For this review, take the finished solid that the model builds, in its own axes (mm). A direction names the side the tool comes from. Give positions to 0.01 mm unless a question says otherwise; leave off trailing zeros. Loops run counter-clockwise (first coordinate to the right, second up) from the corner with the lowest first, then second, coordinate; pieces in that order, holes last. Notation, with made-up numbers: M 65,23.5 L 92,23.5 A32 ccw 92,62.5 Z; hole C -38.75,35.5 d8. An arc over 180 degrees is marked long. Use CSV: the item, a comma, the result in double quotes. Start each with the question number.
1. To check wall thickness, follow line 1 (Y direction, x = 2.75, z = 3.7); line 2 (X direction, y = 0.25, z = 1.6); line 3 (Y direction, x = 3.75, z = 0.95). State the ranges of each line that lie inside material, in increasing order. Write a range as [from, to].
2. Tool access review of faces 1 (the face through (-8, 0, 2)), 2 (the face through (5.1, 5.2, 0)): name each direction out of +Z, -Z, +X, -X, +Y, -Y from which nothing blocks a thin tool from reaching the whole face with its end or side.
3. The part is to be moulded in two halves that separate along X. For faces 3 (the face through (6.834, 7.3, 1.972)), 4 (the face through (4.084, 3.823, 2.125)), 5 (the face through (5.1, 5.2, 4)), say which applies: pulls with the +X half, pulls with the -X half, needs draft (parallel to the pull), parting line crosses it, or undercut.
4. Take a section at B-B, the plane z = 2.9. Write out the cut boundary in (x, y) (3 decimals), and give its area (3 significant figures).
5. Take a section at A-A, the plane z = 0.5. Write out the cut boundary in (x, y) (3 decimals).
6. Insertion check: P1, Ø1.2, axis at y = -8.5, z = 2, coming from the -X side; P2, Ø1, axis at x = -4.5, z = 0.5, coming from the -Y side. Each pin has a flat end and moves straight along its axis. Give the tip position at first contact, or say it passes through.
Autodesk Inventor part; units mm, degrees
ref_plane "YZ Plane" through (0, 0, 0) normal (1, 0, 0) x (0, 1, 0)
ref_plane "XZ Plane" through (0, 0, 0) normal (0, 1, 0) x (-1, 0, 0)
ref_plane "XY Plane" through (0, 0, 0) normal (0, 0, 1) x (1, 0, 0)
sketch "Skizze1" plane through (0, 0, 0) normal (0, 0, 1) x (1, 0, 0)
  circle A0 centre (0, 0) radius 7
  circle A1 centre (0, 0) radius 10
  line L0 (0, 0) -> (-10, 0)
  line L1 (0, 0) -> (0, -10)
  point P0 (0, -7)
  point P1 (-7, 0)
  dimension "d0" = 14
  dimension "d1" = 20
extrude "Extrusion1" add sketch "Skizze1" along normal blind 4 contours A0 L0 A1 L1 picked at (-8.8353, 1.3561)
sketch "Skizze2" plane through (-10, 0, 0) normal (0, -1, 0) x (1, 0, 0)
  line L0 (3, 0) -> (3, 4) construction
  line L1 (3, 2) -> (4.5, 2) construction
  line L2 (4.5, 2) -> (3, 4)
  line L3 (20, 4) -> (0, 4)
  line L4 (4.5, 2) -> (3, 0)
  line L5 (3, 0) -> (3, 4)
  line L6 (10, -0.8) -> (10, 4.8)
  point P0 (10, 0)
  point P1 (10, 4)
  dimension "d4" = 1.5
revolve "Umdrehung1" add sketch "Skizze2" angle 270 about axis through (0, 0, -10) along (0, 0, -1)
properties part number "C-ClipV1"
Result set:
1,line 1,"[-9.61, -6.19], [6.19, 9.61]"
1,line 2,"[-10, -5.79], [5.79, 10]"
1,line 3,"[-9.27, -5.05], [5.05, 9.27]"
2,face 1,"+Z, -Z, -X, -Y"
2,face 2,"-Z, +X, -X, +Y, -Y"
3,face 3,"parting line crosses it"
3,face 4,"undercut"
3,face 5,"needs draft"
4,outline,"M -10,0 L -6.175,0 A6.175 cw long 0,-6.175 L 0,-10 A10 ccw long Z"
4,area,"146 mm2"
5,outline,"M -10,0 L -6.625,0 A6.625 cw long 0,-6.625 L 0,-10 A10 ccw long Z"
6,P1,"x = 0"
6,P2,"y = 4.11"
